For this review, take the finished solid that the model builds, in its own axes (mm). Coordinates: 2 decimals unless noted, no trailing zeros. Order: outer loops, then holes, each group sorted by start corner. A loop starts at its lowest first (then second) coordinate and runs counter-clockwise, first axis right, second up. Notation, with made-up numbers: (-39, 65.25) -> (-1, 65.25) arc R28 ccw to (-1, 94.25) -> close; hole circle Ø7 at (43, 47.5). An arc over 180 degrees is marked (long way). Write item = value, one per line. Start each with the question number.
1) Consider section C-C on z = 1.5. Give the boundary of the cut face in (x, y), and give its area (3 significant figures).
2) Consider section A-A on x = 57.15. Give the boundary of the cut face in (y, z) (3 decimals), and give its area (3 significant figures).
3) Wall thickness on probe 1 along X at (y, z) = (45, 2.5); probe 2 along Y at (x, z) = (19.05, -2.65); probe 3 along Y at (x, z) = (61, 2.75): over which ranges is each line inside the solid? List them lowest first. Write a range as [from, to].
4) Consider section B-B on y = 38.1. State how many separate pieces and enclosed holes the cut face has, and give its area (3 significant figures).
from build123d import *

# Parameters (mm, degrees)
SKETCH1_W           = 76.2
SKETCH1_H           = 76.2
SKETCH1_R           = 4.1656
BOSS_EXTRUDE1_DEPTH = 3.175
CUT_EXTRUDE1_START  = -5.0292
SKETCH2_R           = 4.1656
CUT_EXTRUDE1_DEPTH  = 6.0292
CUT_EXTRUDE1_TAPER  = -41


with BuildPart() as part:
    # Sketch1 → Boss-Extrude1 (new body, symmetric)
    with BuildSketch(Plane.XY):
        with Locations((38.1, 38.1)):
            Rectangle(SKETCH1_W, SKETCH1_H)
        with Locations((19.05, 38.1)):
            Circle(SKETCH1_R, mode=Mode.SUBTRACT)
        with Locations((57.15, 38.1)):
            Circle(SKETCH1_R, mode=Mode.SUBTRACT)
    extrude(amount=BOSS_EXTRUDE1_DEPTH, both=True)

    # Sketch2 → Cut-Extrude1 (cut, through all)
    with BuildSketch(Plane.XY.offset(3.175).offset(CUT_EXTRUDE1_START)):
        with Locations((19.05, 38.1)):
            Circle(SKETCH2_R)
        with Locations((57.15, 38.1)):
            Circle(SKETCH2_R)
    extrude(amount=CUT_EXTRUDE1_DEPTH, taper=CUT_EXTRUDE1_TAPER, mode=Mode.SUBTRACT)


solid = part.part
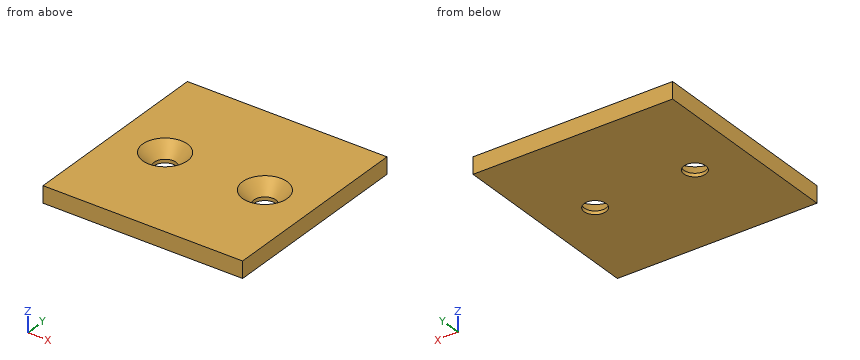
Answer sheet:
q1.outline = (0, 0) -> (76.2, 0) -> (76.2, 76.2) -> (0, 76.2) -> close; hole circle Ø14.16 at (19.05, 38.1); hole circle Ø14.16 at (57.15, 38.1)
q1.area = 5,490 mm2
q2.outline = (0, -3.175) -> (33.934, -3.175) -> (33.934, -1.854) -> (29.563, 3.175) -> (0, 3.175) -> close; (42.266, -3.175) -> (76.2, -3.175) -> (76.2, 3.175) -> (46.637, 3.175) -> (42.266, -1.854) -> close
q2.area = 409 mm2
q3.probe_1 = [0, 15.1], [23, 53.2], [61.1, 76.2]
q3.probe_2 = [0, 33.93], [42.27, 76.2]
q3.probe_3 = [0, 30.9], [45.3, 76.2]
q4.separate_pieces = 3
q4.enclosed_holes = 0
q4.area = 334 mm2
